```python
from build123d import *

# Parameters (mm, degrees)
BOSS_EXTRU_1_DEPTH      = 120
ESQUISSE2_W             = 45
ESQUISSE2_H             = 35
ENL_V_MAT_EXTRU_1_DEPTH = 10
ESQUISSE3_R             = 7
ENL_V_MAT_EXTRU_2_DEPTH = 10
ESQUISSE4_R             = 3
ENL_V_MAT_EXTRU_3_DEPTH = 142.311712183
TROU_TARAUD_M61_D       = 5
TROU_TARAUD_M61_DEPTH   = 15
TROU_TARAUD_M61_TIP     = 1.502151548
ESQUISSE7_W             = 30
ESQUISSE7_H             = 35
ENL_V_MAT_EXTRU_4_DEPTH = 10
ESQUISSE8_R             = 4
ENL_V_MAT_EXTRU_5_DEPTH = 20


with BuildPart() as part:
    # Esquisse1 → Boss.-Extru.1 (new body)
    with BuildSketch(Plane.XY):
        Polygon((0, 0), (0, -40), (-68, -40), (-68, -35), (-5, -35), (-5, 0), align=None)
    extrude(amount=BOSS_EXTRU_1_DEPTH)

    # Esquisse2 → Enlèv. mat.-Extru.1 (cut)
    with BuildSketch(Plane.ZY.offset(5)):
        with Locations((22.5, -17.5)):
            Rectangle(ESQUISSE2_W, ESQUISSE2_H)
        with Locations((97.5, -17.5)):
            Rectangle(ESQUISSE2_W, ESQUISSE2_H)
    extrude(amount=-ENL_V_MAT_EXTRU_1_DEPTH, mode=Mode.SUBTRACT)

    # Esquisse3 → Enlèv. mat.-Extru.2 (cut)
    with BuildSketch(Plane.XZ.offset(40)):
        with Locations((-30, 85.5)):
            Circle(ESQUISSE3_R)
    extrude(amount=-ENL_V_MAT_EXTRU_2_DEPTH, mode=Mode.SUBTRACT)

    # Esquisse4 → Enlèv. mat.-Extru.3 (cut, through all)
    with BuildSketch(Plane.ZY.offset(5)):
        with Locations((50, -5)):
            Circle(ESQUISSE4_R)
        with Locations((50, -25)):
            Circle(ESQUISSE4_R)
    extrude(amount=-ENL_V_MAT_EXTRU_3_DEPTH, mode=Mode.SUBTRACT)

    # Trou taraudé M61
    with Locations(Plane(origin=(-37, -40, 5.5), x_dir=(0, 0, -1), z_dir=(0, -1, 0))):
        with Locations((0, 0), (0, 24)):
            Hole(TROU_TARAUD_M61_D / 2, depth=TROU_TARAUD_M61_DEPTH)
            with Locations((0, 0, -(TROU_TARAUD_M61_DEPTH + TROU_TARAUD_M61_TIP / 2))):  # 118° drill point
                Cone(0, TROU_TARAUD_M61_D / 2, TROU_TARAUD_M61_TIP, mode=Mode.SUBTRACT)

    # Esquisse7 → Enlèv. mat.-Extru.4 (cut)
    with BuildSketch(Plane.ZY.offset(5)):
        with Locations((60, -17.5)):
            Rectangle(ESQUISSE7_W, ESQUISSE7_H)
    extrude(amount=-ENL_V_MAT_EXTRU_4_DEPTH, mode=Mode.SUBTRACT)

    # Esquisse8 → Enlèv. mat.-Extru.5 (cut)
    with BuildSketch(Plane(origin=(0, -35, 0), x_dir=(1, 0, 0), z_dir=(0, 1, 0))):
        with Locations(Location((-20, -33.5, 0), (0, 0, 270))):
            Circle(ESQUISSE8_R)
    extrude(amount=-ENL_V_MAT_EXTRU_5_DEPTH, mode=Mode.SUBTRACT)


solid = part.part
```
Verification items for the finished model (mm, model axes). Give positions to 0.01 mm unless a question says otherwise; leave off trailing zeros. Loops run counter-clockwise (first coordinate to the right, second up) from the corner with the lowest first, then second, coordinate; pieces in that order, holes last.
1. Section check A-A, the plane z = 5.5. Enter the section's corners in (x, y), then the cut area to 3 significant figures.
2. Section check D-D, the plane y = -38.1. Enter the section's corners in (x, z).
3. Mould release check, pull along X, two halves, no side actions. Record for faces 1 (the cylindrical face through (-17.3, -37.47, 30.55)), 2 (the flat face through (-34, -37, 0)), 3 (the flat face through (-68, -38, 59)): released by +X, released by -X, zero draft, split by the parting line, or undercut.
4. Section check B-B, the plane x = -20. Enter the section's corners in (y, z).
5. Thickness scan on line 1 (X direction, y = -38.1, z = 5.5); line 2 (X direction, y = -38.8, z = 33.5); line 3 (Z direction, x = -35, y = -38.3). Record the ranges inside material, lowest first.
6. Section check C-C, the plane z = 33.5. Enter the section's corners in (x, y), then the cut area to 3 significant figures.
Geometry says:
1. outline: (-68, -40) - (-39.5, -40) - (-39.5, -35) - (-68, -35) - close; (-34.5, -40) - (-15.5, -40) - (-15.5, -35) - (-34.5, -35) - close; (-10.5, -40) - (0, -40) - (0, -35) - (-10.5, -35) - close
1. area: 290 mm2
2. outline: (-68, 0) - (0, 0) - (0, 120) - (-68, 120) - close; hole circle Ø5 at (-37, 5.5); hole circle Ø14 at (-30, 85.5); hole circle Ø8 at (-20, 33.5); hole circle Ø5 at (-13, 5.5)
3. face 1: undercut
3. face 2: zero draft
3. face 3: released by -X
4. outline: (-40, 0) - (-35, 0) - (-35, 29.5) - (-40, 29.5) - close; (-40, 37.5) - (-35, 37.5) - (-35, 120) - (-40, 120) - close
5. line 1: x = -68 to -39.5, -34.5 to -15.5, -10.5 to 0
5. line 2: x = -68 to -24, -16 to 0
5. line 3: z = 0 to 4, 7 to 80.6, 90.4 to 120
6. outline: (-68, -40) - (-24, -40) - (-24, -35) - (-68, -35) - close; (-16, -40) - (0, -40) - (0, -35) - (-16, -35) - close
6. area: 300 mm2
